```python
from build123d import *

# Parameters (mm, degrees)
SKETCH1_W                      = 8
SKETCH1_H                      = 1.4
BOSS_EXTRUDE1_DEPTH            = 1
SKETCH2_W                      = 34.6
SKETCH2_H                      = 58
BOSS_EXTRUDE2_DEPTH            = 24
SKETCH3_W                      = 26
SKETCH3_H                      = 55
BOSS_EXTRUDE3_DEPTH            = 1
BOSS_EXTRUDE4_DEPTH            = 1
SKETCH5_W                      = 8
SKETCH5_H                      = 1.4
BOSS_EXTRUDE5_DEPTH            = 1
SKETCH6_W                      = 10.2
SKETCH6_H                      = 8.5
CUT_EXTRUDE1_DEPTH             = 0.1
SKETCH7_W                      = 10.2
SKETCH7_H                      = 8.5
CUT_EXTRUDE2_DEPTH             = 0.1
SKETCH8_W                      = 25
SKETCH8_H                      = 58
BOSS_EXTRUDE6_DEPTH            = 8.4
SKETCH9_W                      = 10
SKETCH9_H                      = 0.9
BOSS_EXTRUDE7_DEPTH            = 1.5
SKETCH10_W                     = 10
SKETCH10_H                     = 0.9
BOSS_EXTRUDE8_DEPTH            = 1.5
SKETCH11_W                     = 12
SKETCH11_H                     = 11.2
CUT_EXTRUDE3_DEPTH             = 12
SKETCH12_W                     = 1
SKETCH12_H                     = 8.5
BOSS_EXTRUDE9_DEPTH            = 12
SKETCH13_W                     = 12
SKETCH13_H                     = 11.2
CUT_EXTRUDE4_DEPTH             = 12
SKETCH14_W                     = 1
SKETCH14_H                     = 8.5
BOSS_EXTRUDE10_DEPTH           = 12
SKETCH15_W                     = 12
SKETCH15_H                     = 11.2
CUT_EXTRUDE5_DEPTH             = 12
SKETCH16_W                     = 1
SKETCH16_H                     = 8.5
BOSS_EXTRUDE11_DEPTH           = 12
SKETCH17_W                     = 12
SKETCH17_H                     = 11.2
CUT_EXTRUDE6_DEPTH             = 12
SKETCH18_W                     = 1
SKETCH18_H                     = 8.5
BOSS_EXTRUDE12_DEPTH           = 12
CUT_EXTRUDE7_DEPTH             = 22
CUT_EXTRUDE8_DEPTH             = 25
CUT_EXTRUDE9_DEPTH             = 1.9
SKETCH22_W                     = 11.2
SKETCH22_H                     = 31
CUT_EXTRUDE10_DEPTH            = 2
SKETCH23_W                     = 2.5
SKETCH23_H                     = 14
BOSS_EXTRUDE13_DEPTH           = 1
SKETCH24_W                     = 11.2
SKETCH24_H                     = 31
CUT_EXTRUDE11_DEPTH            = 2
SKETCH25_W                     = 2.5
SKETCH25_H                     = 14
BOSS_EXTRUDE14_DEPTH           = 1
CUT_EXTRUDE12_DEPTH            = 22
SKETCH27_W                     = 4
SKETCH27_H                     = 3.1
SKETCH28_W                     = 4
SKETCH28_H                     = 3.1
SKETCH29_W                     = 4
SKETCH29_H                     = 3.1
SKETCH30_W                     = 4
SKETCH30_H                     = 3.1
F_2_0_2_DIAMETER_HOLE1_D       = 2
F_2_0_2_DIAMETER_HOLE1_DEPTH   = 1.5
F_4_5_4_5_DIAMETER_HOLE1_D     = 4.5
F_4_5_4_5_DIAMETER_HOLE1_DEPTH = 0.9
F_4_5_4_5_DIAMETER_HOLE2_D     = 4.5
F_4_5_4_5_DIAMETER_HOLE2_DEPTH = 24


with BuildPart() as part:
    # Sketch1 → Boss-Extrude1 (new body)
    with BuildSketch(Plane(origin=(0, 0, 0), x_dir=(-1, 0, 0), z_dir=(0, 0, -1))):
        with Locations((-9.1, 4.55)):
            Rectangle(SKETCH1_W, SKETCH1_H)
    extrude(amount=-BOSS_EXTRUDE1_DEPTH)

    # Sketch2 → Boss-Extrude2 (add)
    with BuildSketch(Plane(origin=(0, 0, 1), x_dir=(-1, 0, 0), z_dir=(0, 0, -1))):
        with Locations((4.2, -23.75)):
            Rectangle(SKETCH2_W, SKETCH2_H)
    extrude(amount=-BOSS_EXTRUDE2_DEPTH)

    # Sketch3 → Boss-Extrude3 (add)
    with BuildSketch(Plane(origin=(0, 0, 1), x_dir=(-1, 0, 0), z_dir=(0, 0, -1))):
        with Locations((0, -23.75)):
            Rectangle(SKETCH3_W, SKETCH3_H)
    extrude(amount=BOSS_EXTRUDE3_DEPTH)

    # Sketch4 → Boss-Extrude4 (add)
    with BuildSketch(Plane(origin=(0, 0, 1), x_dir=(-1, 0, 0), z_dir=(0, 0, -1))):
        Polygon((5.1, 5.25), (21.5, 5.25), (21.5, -52.75), (5.1, -52.75), (5.1, -51.35), (13.1, -51.35), (13.1, 3.85), (5.1, 3.85), align=None)
    extrude(amount=BOSS_EXTRUDE4_DEPTH)

    # Sketch5 → Boss-Extrude5 (add)
    with BuildSketch(Plane(origin=(0, 0, 1), x_dir=(-1, 0, 0), z_dir=(0, 0, -1))):
        with Locations((-9.1, -52.05)):
            Rectangle(SKETCH5_W, SKETCH5_H)
    extrude(amount=BOSS_EXTRUDE5_DEPTH)

    # Sketch6 → Cut-Extrude1 (cut)
    with BuildSketch(Plane.XY.offset(1)):
        with Locations((0, -0.5)):
            Rectangle(SKETCH6_W, SKETCH6_H)
    extrude(amount=-CUT_EXTRUDE1_DEPTH, mode=Mode.SUBTRACT)

    # Sketch7 → Cut-Extrude2 (cut)
    with BuildSketch(Plane.XY.offset(1)):
        with Locations((0, -47)):
            Rectangle(SKETCH7_W, SKETCH7_H)
    extrude(amount=-CUT_EXTRUDE2_DEPTH, mode=Mode.SUBTRACT)

    # Sketch8 → Boss-Extrude6 (add)
    with BuildSketch(Plane(origin=(13.1, 0, 0), x_dir=(0, 0, -1), z_dir=(1, 0, 0))):
        with Locations((-12.5, -23.75)):
            Rectangle(SKETCH8_W, SKETCH8_H)
    extrude(amount=BOSS_EXTRUDE6_DEPTH)

    # Sketch9 → Boss-Extrude7 (add)
    with BuildSketch(Plane.XZ.offset(51.25)):
        with Locations((0, 0.45)):
            Rectangle(SKETCH9_W, SKETCH9_H)
    extrude(amount=BOSS_EXTRUDE7_DEPTH)

    # Sketch10 → Boss-Extrude8 (add)
    with BuildSketch(Plane(origin=(0, 3.75, 0), x_dir=(-1, 0, 0), z_dir=(0, 1, 0))):
        with Locations((0, 0.45)):
            Rectangle(SKETCH10_W, SKETCH10_H)
    extrude(amount=BOSS_EXTRUDE8_DEPTH)

    # Sketch11 → Cut-Extrude3 (cut)
    with BuildSketch(Plane(origin=(0, 5.25, 0), x_dir=(-1, 0, 0), z_dir=(0, 1, 0))):
        with Locations((-12.5, 19.4)):
            Rectangle(SKETCH11_W, SKETCH11_H)
    extrude(amount=-CUT_EXTRUDE3_DEPTH, mode=Mode.SUBTRACT)

    # Sketch12 → Boss-Extrude9 (add)
    with BuildSketch(Plane(origin=(6.5, 0, 0), x_dir=(0, 0, -1), z_dir=(1, 0, 0))):
        with Locations((-14.3, -1.75)):
            Rectangle(SKETCH12_W, SKETCH12_H)
    extrude(amount=BOSS_EXTRUDE9_DEPTH)

    # Sketch13 → Cut-Extrude4 (cut)
    with BuildSketch(Plane(origin=(0, 5.25, 0), x_dir=(-1, 0, 0), z_dir=(0, 1, 0))):
        with Locations((12.5, 19.4)):
            Rectangle(SKETCH13_W, SKETCH13_H)
    extrude(amount=-CUT_EXTRUDE4_DEPTH, mode=Mode.SUBTRACT)

    # Sketch14 → Boss-Extrude10 (add)
    with BuildSketch(Plane(origin=(-18.5, 0, 0), x_dir=(0, 0, -1), z_dir=(1, 0, 0))):
        with Locations((-14.3, -1.75)):
            Rectangle(SKETCH14_W, SKETCH14_H)
    extrude(amount=BOSS_EXTRUDE10_DEPTH)

    # Sketch15 → Cut-Extrude5 (cut)
    with BuildSketch(Plane.XZ.offset(52.75)):
        with Locations((12.5, 19.4)):
            Rectangle(SKETCH15_W, SKETCH15_H)
    extrude(amount=-CUT_EXTRUDE5_DEPTH, mode=Mode.SUBTRACT)

    # Sketch16 → Boss-Extrude11 (add)
    with BuildSketch(Plane.ZY.offset(-18.5)):
        with Locations((14.3, -45.75)):
            Rectangle(SKETCH16_W, SKETCH16_H)
    extrude(amount=BOSS_EXTRUDE11_DEPTH)

    # Sketch17 → Cut-Extrude6 (cut)
    with BuildSketch(Plane.XZ.offset(52.75)):
        with Locations((-12.5, 19.4)):
            Rectangle(SKETCH17_W, SKETCH17_H)
    extrude(amount=-CUT_EXTRUDE6_DEPTH, mode=Mode.SUBTRACT)

    # Sketch18 → Boss-Extrude12 (add)
    with BuildSketch(Plane.ZY.offset(6.5)):
        with Locations((14.3, -45.75)):
            Rectangle(SKETCH18_W, SKETCH18_H)
    extrude(amount=BOSS_EXTRUDE12_DEPTH)

    # Sketch19 → Cut-Extrude7 (cut)
    with BuildSketch(Plane.XY.offset(25)):
        with BuildLine():
            Line((4.25, -52.75), (4.25, -47.5))
            ThreePointArc((4.25, -47.5), (0, -43.25), (-4.25, -47.5))
            Line((-4.25, -47.5), (-4.25, -52.75))
            Line((-4.25, -52.75), (4.25, -52.75))
        make_face()
    extrude(amount=-CUT_EXTRUDE7_DEPTH, mode=Mode.SUBTRACT)

    # Sketch20 → Cut-Extrude8 (cut, through all)
    with BuildSketch(Plane(origin=(0, 0, 1), x_dir=(-1, 0, 0), z_dir=(0, 0, -1))):
        with BuildLine():
            Line((-2.25, -52.75), (2.25, -52.75))
            Line((2.25, -52.75), (2.25, -47.5))
            ThreePointArc((2.25, -47.5), (0, -45.25), (-2.25, -47.5))
            Line((-2.25, -47.5), (-2.25, -52.75))
        make_face()
    extrude(amount=-CUT_EXTRUDE8_DEPTH, mode=Mode.SUBTRACT)

    # Sketch21 → Cut-Extrude9 (cut, through all)
    with BuildSketch(Plane.XY.offset(0.9)):
        with BuildLine():
            Line((-2.25, -52.75), (2.25, -52.75))
            Line((2.25, -52.75), (2.25, -47.5))
            ThreePointArc((2.25, -47.5), (0, -45.25), (-2.25, -47.5))
            Line((-2.25, -47.5), (-2.25, -52.75))
        make_face()
    extrude(amount=-CUT_EXTRUDE9_DEPTH, mode=Mode.SUBTRACT)

    # Sketch22 → Cut-Extrude10 (cut)
    with BuildSketch(Plane(origin=(21.5, 0, 0), x_dir=(0, 0, -1), z_dir=(1, 0, 0))):
        with Locations((-19.4, -23.75)):
            Rectangle(SKETCH22_W, SKETCH22_H)
    extrude(amount=-CUT_EXTRUDE10_DEPTH, mode=Mode.SUBTRACT)

    # Sketch23 → Boss-Extrude13 (add)
    with BuildSketch(Plane(origin=(19.5, 0, 0), x_dir=(0, 0, -1), z_dir=(1, 0, 0))):
        with Locations((-23.75, -23.75)):
            Rectangle(SKETCH23_W, SKETCH23_H)
    extrude(amount=BOSS_EXTRUDE13_DEPTH)

    # Sketch24 → Cut-Extrude11 (cut)
    with BuildSketch(Plane.ZY.offset(21.5)):
        with Locations((19.4, -23.75)):
            Rectangle(SKETCH24_W, SKETCH24_H)
    extrude(amount=-CUT_EXTRUDE11_DEPTH, mode=Mode.SUBTRACT)

    # Sketch25 → Boss-Extrude14 (add)
    with BuildSketch(Plane.ZY.offset(19.5)):
        with Locations((23.75, -23.75)):
            Rectangle(SKETCH25_W, SKETCH25_H)
    extrude(amount=BOSS_EXTRUDE14_DEPTH)

    # Sketch26 → Cut-Extrude12 (cut)
    with BuildSketch(Plane.XY.offset(25)):
        with BuildLine():
            Line((-4.25, 5.25), (-4.25, 0))
            ThreePointArc((-4.25, 0), (0, -4.25), (4.25, 0))
            Line((4.25, 0), (4.25, 5.25))
            Line((4.25, 5.25), (-4.25, 5.25))
        make_face()
    extrude(amount=-CUT_EXTRUDE12_DEPTH, mode=Mode.SUBTRACT)

    # Sketch27 → Revolve1 (revolve)
    with BuildSketch(Plane.XZ.offset(45.75)):
        with Locations((14.5, 16.35)):
            Rectangle(SKETCH27_W, SKETCH27_H)
    revolve(axis=Axis((12.5, -45.75, 17.9), (0, 0, -1)))

    # Sketch28 → Revolve2 (revolve)
    with BuildSketch(Plane.XZ.offset(1.75)):
        with Locations((14.5, 16.35)):
            Rectangle(SKETCH28_W, SKETCH28_H)
    revolve(axis=Axis((12.5, -1.75, 17.9), (0, 0, -1)))

    # Sketch29 → Revolve3 (revolve)
    with BuildSketch(Plane.XZ.offset(45.75)):
        with Locations((-10.5, 16.35)):
            Rectangle(SKETCH29_W, SKETCH29_H)
    revolve(axis=Axis((-12.5, -45.75, 17.9), (0, 0, -1)))

    # Sketch30 → Revolve4 (revolve)
    with BuildSketch(Plane.XZ.offset(1.75)):
        with Locations((-10.5, 16.35)):
            Rectangle(SKETCH30_W, SKETCH30_H)
    revolve(axis=Axis((-12.5, -1.75, 17.9), (0, 0, -1)))

    # Ø2.0 (2) Diameter Hole1
    with Locations(Plane.XY.offset(25)):
        with Locations((12.5, -30)):
            Hole(F_2_0_2_DIAMETER_HOLE1_D / 2, depth=F_2_0_2_DIAMETER_HOLE1_DEPTH)

    # Ø4.5 (4.5) Diameter Hole1
    with Locations(Plane(origin=(0, 0, 0), x_dir=(-1, 0, 0), z_dir=(0, 0, -1))):
        with Locations((0, 0)):
            Hole(F_4_5_4_5_DIAMETER_HOLE1_D / 2, depth=F_4_5_4_5_DIAMETER_HOLE1_DEPTH)

    # Ø4.5 (4.5) Diameter Hole2
    with Locations(Plane(origin=(0, 0, 1), x_dir=(-1, 0, 0), z_dir=(0, 0, -1))):
        with Locations((0, 0)):
            Hole(F_4_5_4_5_DIAMETER_HOLE2_D / 2, depth=F_4_5_4_5_DIAMETER_HOLE2_DEPTH)


solid = part.part
```
Geometry: final body of the model. Coordinates: model frame, mm. A direction names the side the tool comes from. Round coordinates to 2 decimals unless told otherwise and drop trailing zeros. Order: outer loops, then holes, each group sorted by start corner. A loop starts at its lowest first (then second) coordinate and runs counter-clockwise, first axis right, second up. Notation, with made-up numbers: M 73,23 L 118,23 A18 ccw 118,54 Z; hole C -11,-23.75 d8. An arc over 180 degrees is marked long. One line per item, written item: value.
(1) Reachability of faces 1 (the flat face through (-12, -2, 17.9)), 2 (the flat face through (20.5, -24, 24)), 3 (the flat face through (-21, -8.25, 19)), 4 (the flat face through (8, -2, 14.8)) from +Z, -Z, +X, -X, +Y, -Y: full face, straight path, thin tool, end or side. Return the list, or none.
Result sheet:
face 1: +Z, +Y
face 2: +Z, +X
face 3: +Z, -X
face 4: +Z
(2) Cut plane D-D (z = 17). Give the number of separate pieces and of enclosed holes in the cut face, and give its area (3 significant figures).
Result sheet:
separate pieces: 5
enclosed holes: 0
area: 1,850 mm2
(3) Pull-direction query (Y, two-part tool) for faces 5 (the flat face through (2, -46, 3)), 6 (the flat face through (13, -30, 23.5)), 7 (the cylindrical face through (12.63, -29.01, 24.24)); classes: pulls with the +Y half, pulls with the -Y half, needs draft (parallel to the pull), parting line crosses it, or undercut.
Result sheet:
face 5: needs draft
face 6: undercut
face 7: undercut
(4) Cut plane B-B (y = -30). Return the cut outline in (x, z).
Result sheet:
outline: M -21.5,0 L -13.1,0 L -13.1,1 L -13,1 L -13,0 L 13,0 L 13,1 L 13.1,1 L 13.1,0 L 21.5,0 L 21.5,13.8 L 19.5,13.8 L 19.5,22.5 L 20.5,22.5 L 20.5,25 L 13.5,25 L 13.5,23.5 L 11.5,23.5 L 11.5,25 L -20.5,25 L -20.5,22.5 L -19.5,22.5 L -19.5,13.8 L -21.5,13.8 Z
(5) Cut plane C-C (z = 7.25). Return the cut outline in (x, y), and give its area (3 significant figures).
Result sheet:
outline: M -21.5,-52.75 L -4.25,-52.75 L -4.25,-47.5 A4.25 cw 4.25,-47.5 L 4.25,-52.75 L 21.5,-52.75 L 21.5,5.25 L 4.25,5.25 L 4.25,0 A4.25 cw -4.25,0 L -4.25,5.25 L -21.5,5.25 Z
area: 2,350 mm2
(6) Cut plane A-A (x = 0). Return the cut outline in (y, z).
Result sheet:
outline: M -45.25,0 L -2.25,0 L -2.25,0.9 L -4.75,0.9 L -4.75,1 L -2.25,1 L -2.25,3 L -4.25,3 L -4.25,25 L -43.25,25 L -43.25,3 L -45.25,3 L -45.25,1 L -42.75,1 L -42.75,0.9 L -45.25,0.9 Z; M 2.25,0 L 5.25,0 L 5.25,0.9 L 2.25,0.9 Z; M 2.25,1 L 5.25,1 L 5.25,3 L 2.25,3 Z
(7) Line query: probe 1 along X at (y, z) = (-4.5, 20); probe 2 along Y at (x, z) = (12.5, 24.05); probe 3 along Y at (x, z) = (0, 0.35). Output: solid intervals per line, ascending. Write a range as [from, to].
Result sheet:
probe 1: [-21.5, -18.5], [-6.5, 6.5], [18.5, 21.5]
probe 2: [-40.75, -31], [-29, -6.75]
probe 3: [-45.25, -2.25], [2.25, 5.25]
(8) Pin query (flat end, axial travel): P1, Ø1.5, axis at x = 12.5, z = 20, coming from the +Y side; P2, Ø5, axis at y = -32, z = 19, coming from the +X side; P3, Ø3.5, axis at x = -13.5, z = 17.5, coming from the -Y side. Return the tip coordinate at first contact, or that it passes through.
Result sheet:
P1: y = -6.75
P2: x = 19.5
P3: y = -49.75
